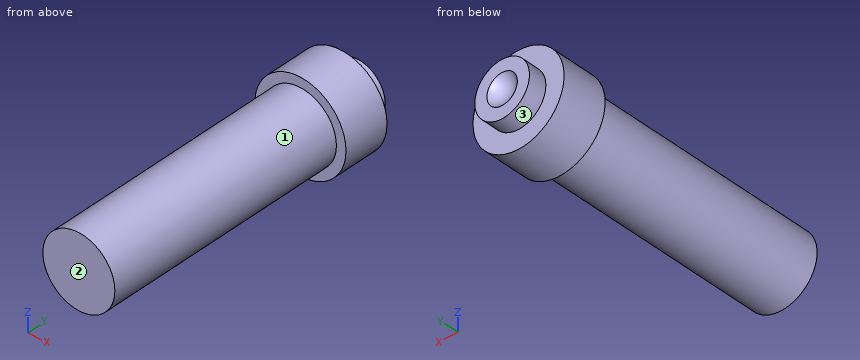
Autodesk Inventor part; units mm, degrees
ref_plane "YZ Plane" through (0, 0, 0) normal (1, 0, 0) x (0, 1, 0)
ref_plane "XZ Plane" through (0, 0, 0) normal (0, 1, 0) x (-1, 0, 0)
ref_plane "XY Plane" through (0, 0, 0) normal (0, 0, 1) x (1, 0, 0)
sketch "Sketch1" plane through (0, 0, 0) normal (0, 1, 0) x (-1, 0, 0)
  circle A0 centre (0, 0) radius 2
  circle A1 centre (0, 0) radius 3
  line L0 (0, 2) -> (0, -2)
  dimension "d0" = 4
  dimension "d1" = 6
extrude "Extrusion1" add sketch "Sketch1" against normal blind 15 contours A0 L0 | L0 A0 | A1
revolve "Revolution1" cut sketch "Sketch1" angle 360 about axis through (0, 0, 2) along (0, 0, -1) picked at (0.2893, 0.6006) contours A0 L0
sketch "Sketch2" plane through (0, 0, 0) normal (0, 1, 0) x (1, 0, 0)
  circle A0 centre (0, 0) radius 3
  circle A1 centre (0, 0) radius 2
extrude "Extrusion2" cut sketch "Sketch2" against normal blind 1.1 contours A0 | A1
sketch "Sketch3" plane through (0, -15, 0) normal (0, -1, 0) x (1, 0, 0)
  circle A0 centre (0, 0) radius 5
  circle A1 centre (0, 0) radius 3
  dimension "d7" = 10
extrude "Extrusion3" add sketch "Sketch3" against normal blind 10
sketch "Sketch4" plane through (0, -15, 0) normal (0, -1, 0) x (1, 0, 0)
  circle A0 centre (0, 0) radius 5
extrude "Extrusion4" cut sketch "Sketch4" against normal blind 5
sketch "Sketch5" plane through (0, -10, 0) normal (0, -1, 0) x (1, 0, 0)
  circle A0 centre (0, 0) radius 3.95
  dimension "d12" = 7.9
extrude "Extrusion5" add sketch "Sketch5" along normal blind 25
sketch "Sketch6" plane through (0, -5, 0) normal (0, 1, 0) x (1, 0, 0)
  circle A0 centre (0, 0) radius 3
  circle A1 centre (0, 0) radius 5
extrude "Extrusion6" cut sketch "Sketch6" against normal blind 0.1
sketch "Sketch7" plane through (0, -10, 0) normal (0, -1, 0) x (1, 0, 0)
  circle A0 centre (0, 0) radius 5
  circle A1 centre (0, 0) radius 3.95
extrude "Extrusion7" add sketch "Sketch7" along normal blind 0.1
sketch "Sketch8" plane through (0, -35, 0) normal (0, -1, 0) x (1, 0, 0)
  circle A0 centre (0, 0) radius 3.95
extrude "Extrusion8" add sketch "Sketch8" along normal blind 0.1
sketch "Sketch9" plane through (0, -5.1, 0) normal (0, 1, 0) x (1, 0, 0)
  circle A0 centre (0, 0) radius 5
extrude "Extrusion9" add sketch "Sketch9" along normal blind 2
sketch "Sketch10" plane through (0, -10.1, 0) normal (0, -1, 0) x (1, 0, 0)
  circle A0 centre (0, 0) radius 5
  circle A1 centre (0, 0) radius 3.95
extrude "Extrusion10" cut sketch "Sketch10" against normal blind 2
properties part number "BARRA"
Check sheet for the modelled part. Datum: model origin and axes. Units: mm. Face numbers are marked on the shaded views. A direction names the side the tool comes from. Round coordinates to 2 decimals unless told otherwise and drop trailing zeros. Order: outer loops, then holes, each group sorted by start corner. A loop starts at its lowest first (then second) coordinate and runs counter-clockwise, first axis right, second up. Notation, with made-up numbers: (69, -26.75) -> (89, -26.75) arc R21 ccw to (89, -20.75) -> close; hole circle Ø9 at (46, 42). An arc over 180 degrees is marked (long way). One line per item, written item: value. Start each with the question number.
Q1. Cross-section at C-C (y = -25). Record the boundary of the cut face in (x, z), and give its area (3 significant figures).
Q2. Cross-section at A-A (x = 0). Record the boundary of the cut face in (y, z), and give its area (3 significant figures).
Q3. Thickness scan on line 1 (Y direction, x = -3.5, z = -0.75); line 2 (X direction, y = -23, z = -0.25); line 3 (Y direction, x = -3.5, z = -2.25). Record the ranges inside material, lowest first.
Q4. Cross-section at B-B (z = 0). Record the boundary of the cut face in (x, y).
Q5. Set-up check for the marked faces 1, 2 and 3: record each of +Z, -Z, +X, -X, +Y, -Y from which the full face is reachable in a straight line by a thin tool's end or side.
Q6. Gauge pin test, flat ends, axial feed: pin 1 Ø4 at (y, z) = (-30, -3) entering from -X; pin 2 Ø6 at (y, z) = (-5.5, -3.5) entering from -X; pin 3 Ø5 at (x, y) = (-2.5, -12.5) entering from -Z. Record the tip position at first contact, or that the pin passes through.
Q7. Cross-section at D-D (z = -2.5). Record the boundary of the cut face in (x, y).
Completed:
1. outline: circle Ø7.9 at (0, 0)
1. area: 49.0 mm²
2. outline: (-35.1, -3.95) -> (-8.1, -3.95) -> (-8.1, -5) -> (-3.1, -5) -> (-3.1, -3) -> (-1.1, -3) -> (-1.1, -1.67) arc R2 cw to (-1.1, 1.67) -> (-1.1, 3) -> (-3.1, 3) -> (-3.1, 5) -> (-8.1, 5) -> (-8.1, 3.95) -> (-35.1, 3.95) -> close
2. area: 273 mm²
3. line 1: y = -35.1 to -3.1
3. line 2: x = -3.94 to 3.94
3. line 3: y = -8.1 to -3.1
4. outline: (-5, -8.1) -> (-3.95, -8.1) -> (-3.95, -35.1) -> (3.95, -35.1) -> (3.95, -8.1) -> (5, -8.1) -> (5, -3.1) -> (3, -3.1) -> (3, -1.1) -> (1.67, -1.1) arc R2 cw to (-1.67, -1.1) -> (-3, -1.1) -> (-3, -3.1) -> (-5, -3.1) -> close
5. face 1: -Y
5. face 2: +Z, -Z, +X, -X, -Y
5. face 3: +Y
6. pin 1: stops at x = -3.82
6. pin 2: stops at x = -4.97
6. pin 3: stops at z = -3.95
7. outline: (-4.33, -8.1) -> (-3.06, -8.1) -> (-3.06, -35.1) -> (3.06, -35.1) -> (3.06, -8.1) -> (4.33, -8.1) -> (4.33, -3.1) -> (1.66, -3.1) -> (1.66, -1.1) -> (-1.66, -1.1) -> (-1.66, -3.1) -> (-4.33, -3.1) -> close
